Verification items for the finished model (mm, model axes). Face numbers are marked on the shaded views. Coordinates: 2 decimals unless noted, no trailing zeros. Answer in a Markdown table with one row per item.
```python
from build123d import *

# Parameters (mm, degrees)
F1_W     = 2.5
F1_H     = 6.85
F3_R     = 12.7
F3_R_2   = 11
F4_DEPTH = 2


# Not quite as in the source:
# - a feature names something its author has since deleted; it is built from what else it names


with BuildPart() as f2:
    # F1 (on Front) → F2 (revolve)
    with BuildSketch(Plane.XZ):
        Polygon((0, 33.3265457083), (0, 11), (7.5, 11), (10, 11), (10, 16), (9.8575705779, 16.2527326282), (9.8575705779, 16.7527326282), (9.5676420315, 16.7549036012), (9.5676420315, 17.2549036012), (9.2777134851, 17.2570745741), (9.2777134851, 17.7570745741), (8.9877849387, 17.759245547), (8.9877849387, 18.259245547), (8.6978563922, 18.26141652), (8.6978563922, 18.76141652), (8.4079278458, 18.7635874929), (8.4079278458, 19.2635874929), (8.1179992994, 19.2657584659), (8.1179992994, 19.7657584659), (7.828070753, 19.7679294388), (7.828070753, 20.2679294388), (7.5381422066, 20.2701004118), (7.5381422066, 20.7701004118), (7.2482136602, 20.7722713847), (7.2482136602, 21.2722713847), (6.9582851138, 21.2744423577), (6.9582851138, 21.7744423577), (6.6683565674, 21.7766133306), (6.6683565674, 22.2766133306), (6.378428021, 22.2787843035), (6.378428021, 22.7787843035), (6.0884994746, 22.7809552765), (6.0884994746, 23.2809552765), (5.7985709282, 23.2831262494), (5.7985709282, 23.7831262494), (5.5086423818, 23.7852972224), (5.5086423818, 24.2852972224), (5.2187138353, 24.2874681953), (5.2187138353, 24.7874681953), (4.9287852889, 24.7896391683), (4.9287852889, 25.2896391683), (4.6388567425, 25.2918101412), (4.6388567425, 25.7918101412), (4.3489281961, 25.7939811141), (4.3489281961, 26.2939811141), (4.0589996497, 26.2961520871), (4.0589996497, 26.7961520871), (3.7690711033, 26.79832306), (3.7690711033, 27.29832306), (3.4791425569, 27.300494033), (3.4791425569, 27.800494033), (3.1892140105, 27.8026650059), (3.1892140105, 28.3026650059), (2.8992854641, 28.3048359789), (2.8992854641, 28.8048359789), (2.6093569177, 28.8070069518), (2.6093569177, 29.3070069518), (2.3194283713, 29.3091779248), (2.3194283713, 29.8091779248), (2.0294998249, 29.8113488977), (2.0294998249, 30.3113488977), (1.7395712784, 30.3135198706), (1.7395712784, 30.8135198706), (1.449642732, 30.8156908436), (1.449642732, 31.3156908436), (1.1597141856, 31.3178618165), (1.1597141856, 31.8178618165), (0.8697856392, 31.8200327895), (0.8697856392, 32.3200327895), (0.5798570928, 32.3222037624), (0.5798570928, 32.8222037624), (0.2899285464, 32.8243747354), (0.2899285464, 33.3243747354), align=None)
        with Locations((8.75, 7.575)):
            Rectangle(F1_W, F1_H)
    revolve(axis=Axis((0, 0, 0), (1, 0, 0)))

    # F3 (on face) → F4 (cut)
    with BuildSketch(Plane(origin=(0, 0, 0), x_dir=(0, -1, 0), z_dir=(-1, 0, 0))):
        Circle(F3_R)
        Circle(F3_R_2, mode=Mode.SUBTRACT)
    extrude(amount=-F4_DEPTH, mode=Mode.SUBTRACT)


solid = f2.part
```
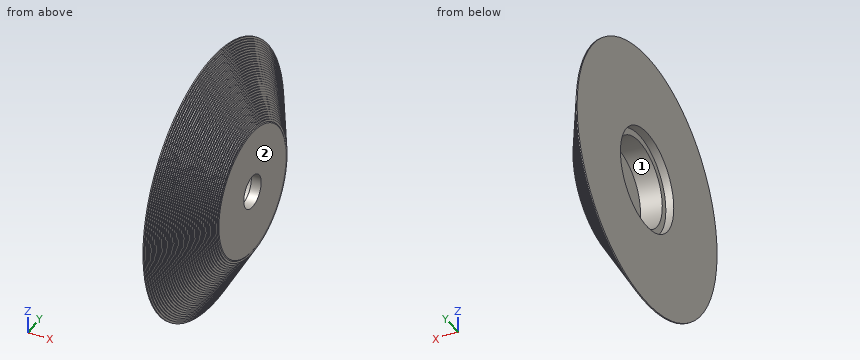
1. Mould release check, pull along Y, two halves, no side actions. Record for the marked faces 1 and 2: released by +Y, released by -Y, zero draft, split by the parting line, or undercut.
Geometry says:
| item | result |
|---|---|
| face 1 | undercut |
| face 2 | zero draft |
2. Thickness scan on line 1 (Y direction, x = 8.2, z = 0); line 2 (Z direction, x = 1, y = 0); line 3 (X direction, y = -22.5, z = -8). Record the ranges inside material, lowest first. Write a range as from..to.
Geometry says:
| item | result |
|---|---|
| line 1 | -19.27..-4.15, 4.15..19.27 |
| line 2 | -31.82..-12.7, 12.7..31.82 |
| line 3 | 0..5.51 |
3. Depth check by flat-ended pin: P1, Ø12, axis at y = 23.5, z = -7.5, coming from the +X side; P2, Ø3, axis at x = 6, y = -15, coming from the +Z side; P3, Ø6.5, axis at y = 4, z = -1, coming from the -X side. Enter the tip coordinate at first touch or a pass-through.
Geometry says:
| item | result |
|---|---|
| P1 | x = 8.7 |
| P2 | z = 21.42 |
| P3 | x = 7.5 |
